Drawing for the job (mm, zero at the part's lowest x, y, z). Round coordinates to 2 decimals unless told otherwise and drop trailing zeros. Order: outer loops, then holes, each group sorted by start corner. A loop starts at its lowest first (then second) coordinate and runs counter-clockwise, first axis right, second up. Notation, with made-up numbers: (72.5, -28.5) - (84.5, -28.5) arc R28 cw to (84.5, -5.5) - close; hole circle Ø9 at (53.25, 49). An arc over 180 degrees is marked (long way). One line per question, with ' | ' between items. Start each with the question number.
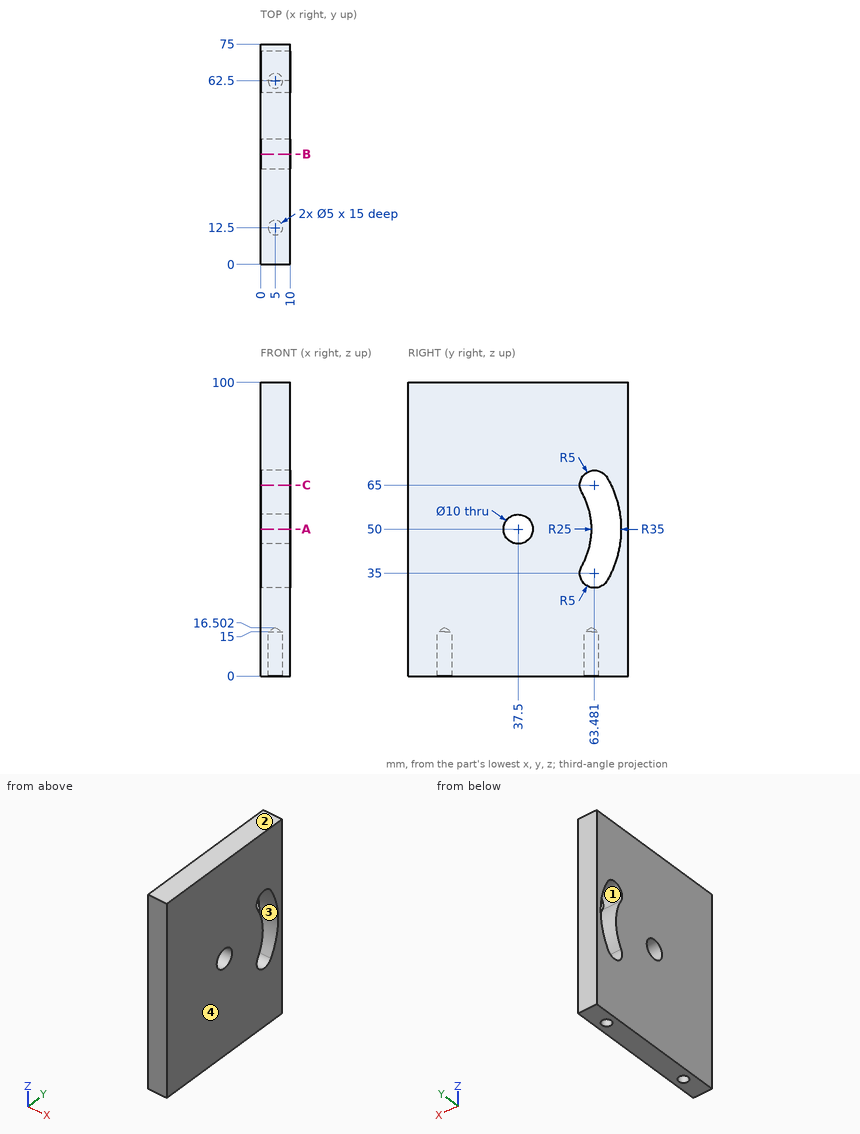
Item 1: Slice it at C-C (z = 65). Write the cut outline in (x, y).
Item 2: Slice it at A-A (z = 50). Write the cut outline in (x, y), plus the area to 3 significant figures.
Item 3: Wall check: line 1 along Y through (x, z) = (5, 10.5); line 2 along Z through (x, y) = (7.5, 37.5); line 3 along X through (y, z) = (62.5, 7). Give the ranges that are in metal, low to high. Write a range as [from, to].
Item 4: Slice it at B-B (y = 37.5). Write the cut outline in (x, z), plus the area to 3 significant figures.
Item 5: Pull direction Z, two halves, no side cores. Call the marked faces 1, 2, 3 and 4: released by +Z, released by -Z, zero draft, split by the parting line, or undercut.
A:
1) outline: (0, 0) - (10, 0) - (10, 58.48) - (0, 58.48) - close; (0, 69.12) - (10, 69.12) - (10, 75) - (0, 75) - close
2) outline: (0, 0) - (10, 0) - (10, 32.5) - (0, 32.5) - close; (0, 42.5) - (10, 42.5) - (10, 62.5) - (0, 62.5) - close; (0, 72.5) - (10, 72.5) - (10, 75) - (0, 75) - close | area: 550 mm^2
3) line 1: [0, 10], [15, 60], [65, 75] | line 2: [0, 45], [55, 100] | line 3: [0, 2.5], [7.5, 10]
4) outline: (0, 0) - (10, 0) - (10, 45) - (0, 45) - close; (0, 55) - (10, 55) - (10, 100) - (0, 100) - close | area: 900 mm^2
5) face 1: undercut | face 2: released by +Z | face 3: undercut | face 4: zero draft
